from build123d import *

# Parameters (mm, degrees)
SKETCH3_R               = 9
BOSS_EXTRUDE1_DEPTH     = 45
CUT_EXTRUDE1_DEPTH      = 14.617013191
CUT_EXTRUDE1_DEPTH_BACK = 14.617013191
BOSS_EXTRUDE2_DEPTH     = 1.2
CUT_EXTRUDE2_DEPTH      = 1.6
SKETCH8_R               = 1.6
SKETCH8_R_2             = 1.4
CUT_EXTRUDE3_DEPTH      = 2.846805277
CUT_EXTRUDE3_DEPTH_BACK = 49.445593418
CUT_EXTRUDE4_DEPTH      = 47.846805277


with BuildPart() as part:
    # Sketch3 → Boss-Extrude1 (new body)
    with BuildSketch(Plane(origin=(-20.344467381, 196.178792599, 0), x_dir=(-0.994665758, -0.103150523, 0), z_dir=(0.103150523, -0.994665758, 0))):
        with Locations((-10.431405186, 0)):
            Circle(SKETCH3_R)
    extrude(amount=BOSS_EXTRUDE1_DEPTH)

    # Sketch4 → Cut-Extrude1 (cut, two sides)
    with BuildSketch(Plane(origin=(10.375761543, 1.076004901, 0), x_dir=(0.103150523, -0.994665758, 0), z_dir=(-0.994665758, -0.103150523, 0))) as cut_extrude1_sk:
        Polygon((-197.230869842, 0), (-188.230869842, 9), (-197.230869842, 9), align=None)
        Polygon((-161.230869842, 9), (-152.230869842, 9), (-152.230869842, 0), align=None)
    extrude(amount=CUT_EXTRUDE1_DEPTH, mode=Mode.SUBTRACT)
    extrude(cut_extrude1_sk.sketch, amount=-CUT_EXTRUDE1_DEPTH_BACK, mode=Mode.SUBTRACT)

    # Sketch5 → Boss-Extrude2 (add, symmetric)
    with BuildSketch(Plane(origin=(10.375761543, 1.076004901, 0), x_dir=(0.103150523, -0.994665758, 0), z_dir=(-0.994665758, -0.103150523, 0))):
        with BuildLine():
            Line((-152.230869842, 0), (-154.210768829, 1.979898987))
            ThreePointArc((-154.210768829, 1.979898987), (-151.865396504, 2.776045612), (-149.805998711, 1.4))
            Line((-149.805998711, 1.4), (-152.230869842, -2.8))
            Line((-152.230869842, -2.8), (-152.230869842, 0))
        make_face()
    extrude(amount=BOSS_EXTRUDE2_DEPTH, both=True)

    # Sketch7 → Cut-Extrude2 (cut, symmetric)
    with BuildSketch(Plane(origin=(10.375761543, 1.076004901, 0), x_dir=(0.103150523, -0.994665758, 0), z_dir=(-0.994665758, -0.103150523, 0))):
        with BuildLine():
            Line((-194.968128142, 2.2627417), (-197.230869842, 0))
            Line((-197.230869842, 0), (-197.230869842, -3.2))
            ThreePointArc((-197.230869842, -3.2), (-194.274455338, -1.224586984), (-194.968128142, 2.2627417))
        make_face()
    extrude(amount=CUT_EXTRUDE2_DEPTH, both=True, mode=Mode.SUBTRACT)

    # Sketch8 → Cut-Extrude3 (cut, two sides)
    with BuildSketch(Plane(origin=(-20.344467381, 196.178792599, 0), x_dir=(0.994665758, 0.103150523, 0), z_dir=(-0.103150523, 0.994665758, 0))) as cut_extrude3_sk:
        with Locations((6.831405186, 3)):
            Circle(SKETCH8_R)
        with Locations((14.031405186, 3)):
            Circle(SKETCH8_R)
        with Locations((10.431405186, -6)):
            Circle(SKETCH8_R_2)
    extrude(amount=CUT_EXTRUDE3_DEPTH, mode=Mode.SUBTRACT)
    extrude(cut_extrude3_sk.sketch, amount=-CUT_EXTRUDE3_DEPTH_BACK, mode=Mode.SUBTRACT)

    # Sketch9 → Cut-Extrude4 (cut, through all)
    with BuildSketch(Plane(origin=(-15.702693845, 151.418833501, 0), x_dir=(0.994665758, 0.103150523, 0), z_dir=(0.103150523, -0.994665758, 0))):
        with BuildLine():
            Line((6.30829956, -8), (14.554510811, -8))
            ThreePointArc((14.554510811, -8), (10.431405186, -9), (6.30829956, -8))
        make_face()
        with BuildLine():
            Line((14.554510811, 8), (6.30829956, 8))
            ThreePointArc((6.30829956, 8), (10.431405186, 9), (14.554510811, 8))
        make_face()
    extrude(amount=-CUT_EXTRUDE4_DEPTH, mode=Mode.SUBTRACT)


solid = part.part
Read the model definition and answer for the solid it produces. Units are mm, in the model's axes. A direction names the side the tool comes from. Coordinates: 2 decimals unless noted, no trailing zeros. Write each loop counter-clockwise with the first axis right and the second up, starting at its lowest first coordinate (ties: lowest second). Pieces come first, ordered by that corner, then holes. Notation, with made-up numbers: M 13,79.25 L 23,79.25 A37 cw 23,116.25 Z; hole C 76,-29 d7. An arc over 180 degrees is marked long. Use a Markdown table: item, result.
Q1. Determine the mould class of faces 6 (the face through (-5.22, 151.27, -0.67)), 7 (the face through (-6.494, 152.119, 1.284)), 8 (the face through (-9.79, 174.97, -2.39)) for opening direction Z: released by +Z, released by -Z, zero draft, split by the parting line, or undercut.
Answer block:
| item | result |
|---|---|
| face 6 | released by -Z |
| face 7 | zero draft |
| face 8 | undercut |
Q2. The part is cut by section A-A, the plane y = 190.5. Give the number of separate pieces and of enclosed holes in the cut face, then the cut area to 3 significant figures.
Answer block:
| item | result |
|---|---|
| separate pieces | 1 |
| enclosed holes | 2 |
| area | 210 mm2 |
Q3. The part is cut by section C-C, the plane z = -6. Write down the section's boundary in (x, y), then the cut area to 3 significant figures.
Answer block:
| item | result |
|---|---|
| outline | M -16.64,196.56 L -12,151.8 L 1.35,153.19 L -3.3,197.95 Z |
| area | 604 mm2 |
Q4. Straight lines are drawn through the part: L1, parallel to X at y = 161.5, z = -2.5; L2, parallel to X at y = 180.5, z = -3.25; L3, parallel to Z at x = -11.25, y = 175.5. For each, find the intervals that lie inside material, in ascending order. Write a range as [from, to].
Answer block:
| item | result |
|---|---|
| L1 | x = [-14.95, -11.41], [-8.35, -4.17], [-1.11, 2.43] |
| L2 | x = [-16.67, -13.44], [-10.26, -6.2], [-3.02, 0.21] |
| L3 | z = [-8, -4.6], [-1.4, 8] |
Q5. Which of the six approach directions +Z, -Z, +X, -X, +Y, -Y give full straight-line access (tool end or side, diameter ignored) to faces 1 (the face through (-8, 175, 8)), 2 (the face through (-8.215, 195.851, -0.43)), 3 (the face through (-11.397, 195.521, -0.43)), 4 (the face through (-4.107, 152.367, 1.284)), 5 (the face through (-5.31, 152.17, 2.78))?
Answer block:
| item | result |
|---|---|
| face 1 | +Z, +X, -X, +Y, -Y |
| face 2 | none |
| face 3 | +Y |
| face 4 | +Z, +X |
| face 5 | +Z |
Q6. Each of these flat-tipped pins is pushed along its axis until it touches: pin 1 Ø1.5 at (y, z) = (172, 2) entering from -X; pin 2 Ø1 at (x, z) = (-10, 2) entering from -Y; pin 3 Ø5 at (x, y) = (-13, 160.5) entering from +Z. Where does it stop, or does it pass through?
Answer block:
| item | result |
|---|---|
| pin 1 | stops at x = -16.33 |
| pin 2 | stops at y = 153.52 |
| pin 3 | stops at z = 7.9 |
